```python
from build123d import *

# Parameters (mm, degrees)
F0_R     = 38.1
F1_DEPTH = 63.5
F2_R     = 7.292745
F3_DEPTH = 101.6


with BuildPart() as f1:
    # F0 (on Top) → F1 (new body)
    with BuildSketch(Plane.XY):
        Circle(F0_R)
    extrude(amount=F1_DEPTH)

    # F2 (on Top) → F3 (join)
    with BuildSketch(Plane.XY):
        with Locations((6.542289, 24.649761)):
            Circle(F2_R)
        with Locations((-24.618464, -6.659092)):
            Circle(F2_R)
        with Locations((18.076175, -17.990669)):
            Circle(F2_R)
    extrude(amount=F3_DEPTH)


solid = f1.part
```
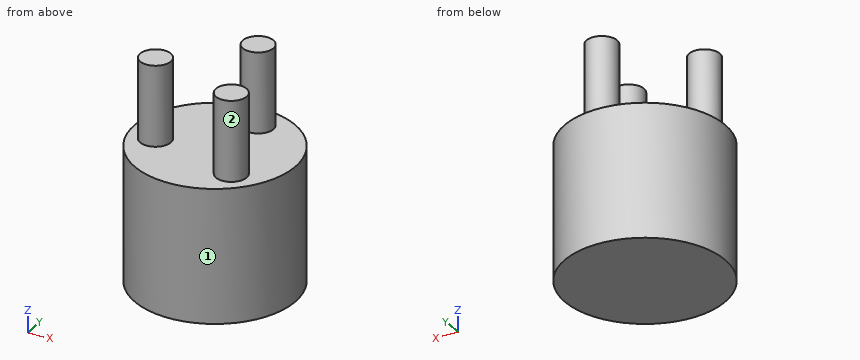
Check sheet for the modelled part. Datum: model origin and axes. Units: mm. Face numbers are marked on the shaded views. A direction names the side the tool comes from. Round coordinates to 2 decimals unless told otherwise and drop trailing zeros. Loops run counter-clockwise (first coordinate to the right, second up) from the corner with the lowest first, then second, coordinate; pieces in that order, holes last. Notation, with made-up numbers: M -28,58.5 L 20,58.5 A32 ccw 20,93.5 Z; hole C 14,-8 d9. An arc over 180 degrees is marked long. Answer as a JSON object with one key per item and string values.
1. Section check A-A (z = 61). Record the boundary of the cut face in (x, y).
Reply:
{"outline": "C 0,0 d76.2"}
2. Section check B-B (x = 6.5). Record the boundary of the cut face in (y, z).
Reply:
{"outline": "M -37.54,0 L 37.54,0 L 37.54,63.5 L 31.94,63.5 L 31.94,101.6 L 17.36,101.6 L 17.36,63.5 L -37.54,63.5 Z"}
3. Gauge pin test, flat ends, axial feed: P1, Ø6, axis at x = -2.5, z = 85.5, coming from the -Y side; P2, Ø4, axis at y = -16.5, z = 56, coming from the -X side; P3, Ø10, axis at y = 23.5, z = 75.5, coming from the +X side. Record the tip position at first contact, or that the pin passes through.
Reply:
{"P1": "stops at y = 20.57", "P2": "stops at x = -35.23", "P3": "stops at x = 13.84"}
4. Section check C-C (z = 74). Record the boundary of the cut face in (x, y), plus the area to 3 significant figures.
Reply:
{"outline": "C -24.62,-6.66 d14.59; C 6.54,24.65 d14.59; C 18.08,-17.99 d14.59", "area": "501 mm²"}
5. Access from +Z, -Z, +X, -X, +Y, -Y to the whole of each face (thin tool, end or side, straight path). Record for the marked faces 1 and 2.
Reply:
{"face 1": "+Z, -Z", "face 2": "+Z"}
6. Section check D-D (y = 13). Record the boundary of the cut face in (x, z), plus the area to 3 significant figures.
Reply:
{"outline": "M -35.81,0 L 35.81,0 L 35.81,63.5 L -35.81,63.5 Z", "area": "4,550 mm²"}
7. Scan lines: line 1 (Z direction, x = 29.5, y = -16); line 2 (Y direction, x = 30, z = 29); line 3 (X direction, y = -20.5, z = 39.5). Record each from-to range of solid material in increasing order.
Reply:
{"line 1": "z = 0 to 63.5", "line 2": "y = -23.49 to 23.49", "line 3": "x = -32.11 to 32.11"}
